The model under review builds one solid part; all positions refer to its coordinate system, in mm. Coordinates: 2 decimals unless noted, no trailing zeros. Order: outer loops, then holes, each group sorted by start corner. A loop starts at its lowest first (then second) coordinate and runs counter-clockwise, first axis right, second up. Notation, with made-up numbers: (-12.5, 37) -> (7.5, 37) arc R16 ccw to (7.5, 47) -> close; hole circle Ø7 at (85, 5). An arc over 180 degrees is marked (long way). Use one line per item in the form item = value. Start each with the question number.
(1) Take a section at D-D (y = 10). State the section outline as (x, z) points, then the cut area to 3 significant figures.
(2) Take a section at C-C (x = 1.55). State the section outline as (y, z) points.
(3) Mouldability with a two-part tool opening along Y and no side actions: class faces 1 (the flat face through (1, 0, 15)), 2 (the flat face through (1, 34.8, 22.6)), 3 (the flat face through (1, 10, 30)), 4 (the cylindrical face through (0.99, 46.42, 6.76)) as +Y half, -Y half, draft (parallel to the pull), parting line (faces both ways), or undercut.
(4) Take a section at A-A (y = 45). State the section outline as (x, z) points, then the cut area to 3 significant figures.
(5) Take a section at B-B (z = 25). State the section outline as (x, y) points.
(6) Wall thickness on line 1 along Y through (x, z) = (1.05, 7.5); line 2 along Y through (x, z) = (0.1, 5); line 3 along Y through (x, z) = (1, 25): over which ranges is each line inside the solid? List them lowest first.
Autodesk Inventor part; units mm, degrees
ref_plane "YZ Plane" through (0, 0, 0) normal (1, 0, 0) x (0, 1, 0)
ref_plane "XZ Plane" through (0, 0, 0) normal (0, 1, 0) x (-1, 0, 0)
ref_plane "XY Plane" through (0, 0, 0) normal (0, 0, 1) x (1, 0, 0)
sketch "スケッチ1" plane through (0, 0, 0) normal (1, 0, 0) x (0, 1, 0)
  line L0 (0, 0) -> (50, 0)
  line L1 (50, 0) -> (50, 15)
  line L2 (50, 15) -> (0, 15) construction
  line L3 (0, 15) -> (0, 0)
  line L4 (0, 0) -> (20, 0)
  line L5 (20, 0) -> (20, 30) construction
  line L6 (20, 30) -> (0, 30)
  line L7 (0, 30) -> (0, 0)
  line L8 (20, 30) -> (50, 15)
  dimension "d0" = 15
  dimension "d1" = 20
  dimension "d2" = 30
  dimension "d3" = 30
extrude "押し出し1" add sketch "スケッチ1" along normal blind 2
sketch "スケッチ2" plane through (2, 0, 0) normal (1, 0, 0) x (0, 0, -1)
  line L0 (-30, 20) -> (-30, 0)
  line L1 (-30, 10) -> (0, 10) construction
  line L2 (0, 0) -> (0, 50)
  line L3 (0, 50) -> (-15, 50)
  line L4 (-7.5, 50) -> (-7.5, 0) construction
  line L5 (-30, 0) -> (0, 0)
  point P0 (-25, 10)
  point P1 (-5, 10)
  point P2 (-7.5, 25)
  point P3 (-7.5, 45)
  dimension "d6" = 20
  dimension "d7" = 5
  dimension "d8" = 20
  dimension "d9" = 5
hole "穴1" at (2, 10, 25) at (2, 10, 5) at (2, 25, 7.5) at (2, 45, 7.5) direction (-1, 0, 0) diameter 3.2 end through all
properties part number "FrameJoint2015" material "アルミニウム 6061"
Findings:
q1.outline = (0, 0) -> (2, 0) -> (2, 3.4) -> (0, 3.4) -> close; (0, 6.6) -> (2, 6.6) -> (2, 23.4) -> (0, 23.4) -> close; (0, 26.6) -> (2, 26.6) -> (2, 30) -> (0, 30) -> close
q1.area = 47.2 mm²
q2.outline = (0, 0) -> (50, 0) -> (50, 15) -> (20, 30) -> (0, 30) -> close; hole circle Ø3.2 at (10, 5); hole circle Ø3.2 at (10, 25); hole circle Ø3.2 at (25, 7.5); hole circle Ø3.2 at (45, 7.5)
q3.face_1 = -Y half
q3.face_2 = +Y half
q3.face_3 = draft
q3.face_4 = undercut
q4.outline = (0, 0) -> (2, 0) -> (2, 5.9) -> (0, 5.9) -> close; (0, 9.1) -> (2, 9.1) -> (2, 17.5) -> (0, 17.5) -> close
q4.area = 28.6 mm²
q5.outline = (0, 0) -> (2, 0) -> (2, 8.4) -> (0, 8.4) -> close; (0, 11.6) -> (2, 11.6) -> (2, 30) -> (0, 30) -> close
q6.line_1 = 0 to 23.4, 26.6 to 43.4, 46.6 to 50
q6.line_2 = 0 to 8.4, 11.6 to 50
q6.line_3 = 0 to 8.4, 11.6 to 30
